from build123d import *

# Parameters (mm, degrees)
F0_R      = 7.62
F1_DEPTH  = 22.86
F2_R      = 5.3975
F3_DEPTH  = 25.4
F4_W      = 17.78
F4_H      = 45.5848994723
F5_DEPTH  = 3.81
F6_DEPTH  = 25.4
F7_R      = 6.0983154317
F8_DEPTH  = 25.4
F9_R      = 3.7193661061
F10_DEPTH = 17.78
F11_DEPTH = 25.4


with BuildPart() as f1:
    # F0 (on Front) → F1 (new body)
    with BuildSketch(Plane.XZ):
        with Locations((-16.9606450945, 18.8963711262)):
            Circle(F0_R)
    extrude(amount=F1_DEPTH)

    # F2 (on face) → F3 (cut)
    with BuildSketch(Plane.XZ.offset(22.86)):
        with Locations((-16.9606450945, 18.8963711262)):
            Circle(F2_R)
    extrude(amount=-F3_DEPTH, mode=Mode.SUBTRACT)

    # F4 (on Front) → F5 (join)
    with BuildSketch(Plane.XZ):
        with Locations((-16.7762902565, 15.3014517855)):
            Rectangle(F4_W, F4_H)
    extrude(amount=-F5_DEPTH)

    # F6 (cut): a face of the model
    f6_faces = [f1.faces().sort_by_distance(p)[0] for p in [
        (-16.9606450945, 0, 18.8963711262),
    ]]
    extrude(f6_faces, amount=-F6_DEPTH, mode=Mode.SUBTRACT)

    # F7 (on face) → F8 (cut)
    with BuildSketch(Plane(origin=(0, 3.81, 0), x_dir=(-1, 0, 0), z_dir=(0, 1, 0))):
        with Locations((16.9606450945, 18.8963711262)):
            Circle(F7_R)
    extrude(amount=-F8_DEPTH, mode=Mode.SUBTRACT)

    # F9 (on Top) → F10 (cut)
    with BuildSketch(Plane.XY):
        with Locations((-17.3269938678, -7.0897382684)):
            Circle(F9_R)
    extrude(amount=F10_DEPTH, mode=Mode.SUBTRACT)

    # F11 (cut): a face of the model
    f11_faces = [f1.faces().sort_by_distance(p)[0] for p in [
        (-11.0348160706, -21.59, 18.8963711262),
    ]]
    extrude(f11_faces, amount=-F11_DEPTH, mode=Mode.SUBTRACT)


solid = f1.part
Check sheet for the modelled part. Datum: model origin and axes. Units: mm. A direction names the side the tool comes from. Coordinates: 2 decimals unless noted, no trailing zeros. Loops run counter-clockwise (first coordinate to the right, second up) from the corner with the lowest first, then second, coordinate; pieces in that order, holes last. Notation, with made-up numbers: (1, 47) -> (24, 47) arc R25 cw to (24, 73) -> close; hole circle Ø3 at (69, -16). An arc over 180 degrees is marked (long way). Answer in a Markdown table with one row per item.
1. Sectioned sample at C-C, the plane x = -21.5. Record the boundary of the cut face in (y, z).
Check values:
| item | result |
|---|---|
| outline | (-22.86, 12.78) -> (0, 12.78) -> (0, -7.49) -> (3.81, -7.49) -> (3.81, 14.82) -> (-22.86, 14.82) -> close; (-22.86, 22.97) -> (3.81, 22.97) -> (3.81, 38.09) -> (0, 38.09) -> (0, 25.02) -> (-22.86, 25.02) -> close |
2. Access from +Z, -Z, +X, -X, +Y, -Y to the whole of each face (thin tool, end or side, straight path). Record for faces 1 (the face through (-12.86, -11.27, 25.32)), 2 (the face through (-17, 3.81, 11)), 3 (the face through (-18.13, -10.72, 12.45)).
Check values:
| item | result |
|---|---|
| face 1 | -Y |
| face 2 | +Z, -Z, +X, -X, +Y |
| face 3 | -Z |
3. Go/stop test with flat-tipped pins: pin 1 (1 mm diameter, centred on y = -11, z = 9, fed in from -X); pin 2 (3 mm diameter, centred on x = -19, y = -14, fed in from -Z); pin 3 (10 mm diameter, centred on y = -19.5, z = 22, fed in from -X); pin 4 (2 mm diameter, centred on y = -18, z = 25.5, fed in from -X). Record where each tip stops, or that it passes through.
Check values:
| item | result |
|---|---|
| pin 1 | passes through |
| pin 2 | stops at z = 11.3 |
| pin 3 | stops at x = -24.58 |
| pin 4 | stops at x = -22.12 |
4. Sectioned sample at A-A, the plane x = -18.75. Record the boundary of the cut face in (y, z), then the cut area to 3 significant figures.
Check values:
| item | result |
|---|---|
| outline | (-22.86, 11.49) -> (-10.53, 11.49) -> (-10.53, 13.07) -> (-22.86, 13.07) -> close; (-22.86, 24.73) -> (3.81, 24.73) -> (3.81, 38.09) -> (0, 38.09) -> (0, 26.3) -> (-22.86, 26.3) -> close; (-3.65, 11.49) -> (0, 11.49) -> (0, -7.49) -> (3.81, -7.49) -> (3.81, 13.07) -> (-3.65, 13.07) -> close |
| area | 191 mm2 |
5. Sectioned sample at B-B, the plane z = 21.5. Record the boundary of the cut face in (x, y).
Check values:
| item | result |
|---|---|
| outline | (-25.67, 0) -> (-24.12, 0) -> (-24.12, -22.86) -> (-22.48, -22.86) -> (-22.48, 3.81) -> (-25.67, 3.81) -> close; (-11.45, -22.86) -> (-9.8, -22.86) -> (-9.8, 0) -> (-7.89, 0) -> (-7.89, 3.81) -> (-11.45, 3.81) -> close |
6. Sectioned sample at D-D, the plane z = -3.5. Record the boundary of the cut face in (x, y).
Check values:
| item | result |
|---|---|
| outline | (-25.67, 0) -> (-7.89, 0) -> (-7.89, 3.81) -> (-25.67, 3.81) -> close |
7. Material ranges on line 1 along Z through (x, y) = (-16.75, 0.5); line 2 along Y through (x, z) = (-15.25, 34); line 3 along Z through (x, y) = (-19, -0.25), recorded low to high. Write a range as [from, to].
Check values:
| item | result |
|---|---|
| line 1 | z = [-7.49, 12.8], [24.99, 38.09] |
| line 2 | y = [0, 3.81] |
| line 3 | z = [11.55, 13.15], [24.64, 26.24] |
8. Release check for a two-part mould opening along Z. For faces 4 (the face through (-17, 0, 11)), 5 (the face through (-17, 2, 38.094)), 6 (the face through (-17, 2, -7.491)), 7 (the face through (-16.167, -9.338, 24.943)) record: released by +Z, released by -Z, zero draft, split by the parting line, or undercut.
Check values:
| item | result |
|---|---|
| face 4 | zero draft |
| face 5 | released by +Z |
| face 6 | released by -Z |
| face 7 | undercut |
